Check sheet for the modelled part. Datum: model origin and axes. Units: mm. A direction names the side the tool comes from. Round coordinates to 2 decimals unless told otherwise and drop trailing zeros. Loops run counter-clockwise (first coordinate to the right, second up) from the corner with the lowest first, then second, coordinate; pieces in that order, holes last. Notation, with made-up numbers: (85.5, -34) - (129.5, -34) arc R26 ccw to (129.5, -1) - close; hole circle Ø10 at (26.25, 48.5). An arc over 180 degrees is marked (long way). Answer in a Markdown table with one row per item. Add a question column.
(1) Cross-section at A-A on z = 21. Enter the section's corners in (x, y), then the cut area to 3 significant figures.
(2) Gauge pin test, flat ends, axial feed: pin 1 (4.5 mm diameter, centred on x = -3.5, z = -6.5, fed in from -Y); pin 2 (1 mm diameter, centred on y = 1, z = 34.5, fed in from +X); pin 3 (4.5 mm diameter, centred on x = 2, z = -7, fed in from -Y). Record the tip position at first contact, or that the pin passes through.
(3) Thickness scan on line 1 along X through (y, z) = (0.25, 17); line 2 along Z through (x, y) = (-0.5, 0.5); line 3 along Y through (x, z) = (-2, -3). Record the ranges inside material, lowest first.
(4) Mould release check, pull along X, two halves, no side actions. Record for faces 4 (the flat face through (1, 3, -5)), 5 (the flat face through (1, -3, -5)), 6 (the cylindrical face through (4.436, -2.307, 12.738)), 7 (the flat face through (3, 1, -5)): +X half, -X half, draft (parallel to the pull), parting line (faces both ways), or undercut.
(5) Access from +Z, -Z, +X, -X, +Y, -Y to the whole of each face (thin tool, end or side, straight path). Record for faces 1 (the flat face through (2, -2, -9.94)), 2 (the flat face through (-1, -3, -5)), 3 (the flat face through (-3, 1, -5)).
from build123d import *

# Parameters (mm, degrees)
F2_W     = 10
F2_H     = 2
F3_DEPTH = 25
F4_W     = 2
F4_H     = 10
F5_DEPTH = 25


with BuildPart() as f1:
    # F0 (on Right) → F1 (revolve)
    with BuildSketch(Plane.YZ):
        with BuildLine():
            Line((0, -9.940476), (0, 40.059524))
            Line((0, 40.059524), (-1, 40.059524))
            ThreePointArc((-1, 40.059524), (-3.828427, 38.887951), (-5, 36.059524))
            Line((-5, 36.059524), (-5, -9.940476))
            Line((-5, -9.940476), (0, -9.940476))
        make_face()
    revolve(axis=Axis((0, 0, 15.059524), (0, 0, -1)))

    # F2 (on Top) → F3 (cut)
    with BuildSketch(Plane.XY):
        Rectangle(F2_W, F2_H)
    extrude(amount=-F3_DEPTH, mode=Mode.SUBTRACT)

    # F4 (on Top) → F5 (cut)
    with BuildSketch(Plane.XY):
        Rectangle(F4_W, F4_H)
    extrude(amount=-F5_DEPTH, mode=Mode.SUBTRACT)


solid = f1.part
Answers:
| question | item | result |
|---|---|---|
| 1 | outline | circle Ø10 at (0, 0) |
| 1 | area | 78.5 mm^2 |
| 2 | pin 1 | stops at y = -4.84 |
| 2 | pin 2 | stops at x = 4.97 |
| 2 | pin 3 | stops at y = -4.9 |
| 3 | line 1 | x = -4.99 to 4.99 |
| 3 | line 2 | z = 0 to 40.06 |
| 3 | line 3 | y = -4.58 to -1, 1 to 4.58 |
| 4 | face 4 | undercut |
| 4 | face 5 | undercut |
| 4 | face 6 | parting line |
| 4 | face 7 | draft |
| 5 | face 1 | -Z, +X, -X, +Y, -Y |
| 5 | face 2 | -Z, +Y, -Y |
| 5 | face 3 | -Z, +X, -X |
